```python
from build123d import *

# Parameters (mm, degrees)
ESQUISSE3_R             = 2.15
ENL_V_MAT_EXTRU_1_DEPTH = 85.070480268
ESQUISSE4_W             = 1.2
ESQUISSE4_H             = 7.846267026
BOSS_EXTRU_1_DEPTH      = 6.35


with BuildPart() as part:
    # Esquisse1 → Révolution1 (revolve)
    with BuildSketch(Plane.XY):
        with BuildLine():
            Line((3.96875, 0), (3.96875, 9.534696006))
            ThreePointArc((3.96875, 9.534696006), (5.270377511, 15.960075858), (8.970022713, 21.372318074))
            Line((8.970022713, 21.372318074), (39.238684771, 50.8))
            Line((39.238684771, 50.8), (38.1, 50.8))
            Line((38.1, 50.8), (8.176272713, 21.707669228))
            ThreePointArc((8.176272713, 21.707669228), (4.476627511, 16.295427012), (3.175, 9.87004716))
            Line((3.175, 9.87004716), (3.175, 0))
            Line((3.175, 0), (3.96875, 0))
        make_face()
    revolve(axis=Axis((0, 0, 0), (0, 1, 0)))

    # Esquisse2 → Révolution2 (revolve)
    with BuildSketch(Plane.XY, mode=Mode.PRIVATE) as r_volution2_sk:
        Polygon((39.238684771, 50.8), (47.366684771, 50.8), (47.366684771, 47.625), (35.97295007, 47.625), align=None)
    revolve(r_volution2_sk.sketch.rotate(Axis((0, 0, 0), (0, 1, 0)), 180), axis=Axis((0, 0, 0), (0, 1, 0)))

    # Esquisse3 → Enlèv. mat.-Extru.1 (cut, through all)
    with BuildSketch(Plane(origin=(0, 50.8, 0), x_dir=(1, 0, 0), z_dir=(0, 1, 0))):
        with Locations(Location((0, -42.794684771, 0), (0, 0, 180))):
            Circle(ESQUISSE3_R)
        with Locations(Location((-42.53639594, -4.694684771, 0), (0, 0, 180))):
            Circle(ESQUISSE3_R)
        with Locations(Location((42.53639594, -4.694684771, 0), (0, 0, 180))):
            Circle(ESQUISSE3_R)
    extrude(amount=-ENL_V_MAT_EXTRU_1_DEPTH, mode=Mode.SUBTRACT)

    # Esquisse4 → Boss.-Extru.1 (add)
    with BuildSketch(Plane.XZ):
        Rectangle(ESQUISSE4_W, ESQUISSE4_H)
    extrude(amount=-BOSS_EXTRU_1_DEPTH)


solid = part.part
```
Could you check a few things on this model? Use its own coordinates, in mm. A direction names the side the tool comes from. Give positions to 0.01 mm unless a question says otherwise; leave off trailing zeros. Order: outer loops, then holes, each group sorted by start corner. A loop starts at its lowest first (then second) coordinate and runs counter-clockwise, first axis right, second up.
Q1. I'm going to push flat-ended pins straight in: P1, Ø4, axis at x = 18.5, z = -20.5, coming from the +Y side; P2, Ø1, axis at x = 20, y = 35, coming from the -Z side; P3, Ø10, axis at y = 10.5, z = -7.5, coming from the -X side; P4, Ø3, axis at y = 23.5, z = 16, coming from the +X side. Where does each tip first touch, or does it pass through?
Q2. Suppose I cut it at A-A, the plane z = 0. Write out the boundary of the cut face in (x, y) (3 decimals), and give its area (3 significant figures).
Q3. Suppose I cut it at C-C, the plane y = 41.5. Write out the boundary of the cut face in (x, z), and give its area (3 significant figures).
Q4. If I drill on line 1 along X through (y, z) = (3.25, 0) (3 decimals); line 2 along Z through (x, y) = (0, 6.5) (3 decimals); line 3 along Y through (x, z) = (36, -23) (3 decimals), over which ranges is the centre line in solid material (lowest first)?
Q5. Suppose I cut it at B-B, the plane y = 32. Write out the boundary of the cut face in (x, z).
Q6. We'd pull the mould along Z, two halves only. Please class faces 4 (the flat face through (-32, 50.8, 21)), 5 (the conical face through (-2.311, 23.015, 10.406)), 6 (the cylindrical face through (44.684, 49.235, 4.789)): +Z half, -Z half, draft (parallel to the pull), parting line (faces both ways), or undercut.
Q7. For faces 1 (the flat face through (0.6, 3, 0)), 2 (the cylindrical face through (-0.86, 4.834, 3.874)), 3 (the flat face through (0, 0, 0)), which set-ups out of +Z, -Z, +X, -X, +Y, -Y let a thin tool reach every point of the face, with its end or its side?
Solution:
1. P1: stops at y = 42.55
1. P2: stops at z = -12.63
1. P3: stops at x = -3.15
1. P4: passes through
2. outline: (-47.367, 47.625) - (-35.973, 47.625) - (-8.97, 21.372) arc R16.51 cw to (-3.969, 9.535) - (-3.969, 0) - (-3.175, 0) - (-3.175, 9.87) arc R16.51 ccw to (-8.176, 21.708) - (-38.1, 50.8) - (-47.367, 50.8) - close; (-0.6, 0) - (0.6, 0) - (0.6, 6.35) - (-0.6, 6.35) - close; (3.175, 0) - (3.969, 0) - (3.969, 9.535) arc R16.51 cw to (8.97, 21.372) - (35.973, 47.625) - (47.367, 47.625) - (47.367, 50.8) - (38.1, 50.8) - (8.176, 21.708) arc R16.51 ccw to (3.175, 9.87) - close
2. area: 174 mm2
3. outline: circle Ø59.35 at (0, 0); hole circle Ø57.07 at (0, 0)
3. area: 208 mm2
4. line 1: x = -3.969 to -3.175, -0.6 to 0.6, 3.175 to 3.969
4. line 2: z = -3.969 to -3.175, 3.175 to 3.969
4. line 3: y = 47.625 to 50.8
5. outline: circle Ø39.8 at (0, 0); hole circle Ø37.53 at (0, 0)
6. face 4: draft
6. face 5: parting line
6. face 6: undercut
7. face 1: +Y, -Y
7. face 2: -Y
7. face 3: +Z, -Z, +X, -X, -Y
